Geometry: final body of the model. Coordinates: model frame, mm. Face numbers are marked on the shaded views. Round coordinates to 2 decimals unless told otherwise and drop trailing zeros. Loops run counter-clockwise (first coordinate to the right, second up) from the corner with the lowest first, then second, coordinate; pieces in that order, holes last. Notation, with made-up numbers: M 58,15 L 83,15 A31 ccw 83,52 Z; hole C 72,18.25 d11. An arc over 180 degrees is marked long. Return JSON: item names as keys, results as strings.
from build123d import *

# Parameters (mm, degrees)
CROQUIS1_R              = 32
SALIENTE_EXTRUIR1_DEPTH = 5
CROQUIS2_R              = 1.25
CORTAR_EXTRUIR1_DEPTH   = 46.530209751


with BuildPart() as part:
    # Croquis1 → Saliente-Extruir1 (new body)
    with BuildSketch(Plane.XY):
        Circle(CROQUIS1_R)
    extrude(amount=SALIENTE_EXTRUIR1_DEPTH)

    # Croquis2 → Cortar-Extruir1 (cut, through all)
    with BuildSketch(Plane.XY.offset(5)):
        with Locations((0, 28)):
            Circle(CROQUIS2_R)
        with Locations((19.798989873, 19.798989873)):
            Circle(CROQUIS2_R)
        with Locations((28, 0)):
            Circle(CROQUIS2_R)
        with Locations((19.798989873, -19.798989873)):
            Circle(CROQUIS2_R)
        with Locations((0, -28)):
            Circle(CROQUIS2_R)
        with Locations((-19.798989873, -19.798989873)):
            Circle(CROQUIS2_R)
        with Locations((-28, 0)):
            Circle(CROQUIS2_R)
        with Locations((-19.798989873, 19.798989873)):
            Circle(CROQUIS2_R)
    extrude(amount=-CORTAR_EXTRUIR1_DEPTH, mode=Mode.SUBTRACT)


solid = part.part
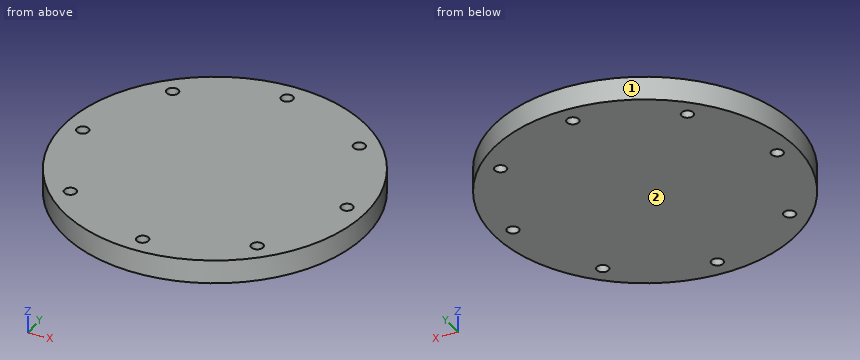
Q1. Section query D-D (x = 28). Output: boundary loops of the cut face in (y, z).
Determined:
{"outline": "M -15.49,0 L -1.25,0 L -1.25,5 L -15.49,5 Z; M 1.25,0 L 15.49,0 L 15.49,5 L 1.25,5 Z"}
Q2. Pin query (flat end, axial travel): pin 1 (2 mm diameter, centred on y = 25, z = 2, fed in from +X); pin 2 (2 mm diameter, centred on x = -22, z = 4, fed in from -Y); pin 3 (1 mm diameter, centred on x = 20, z = 2.5, fed in from -Y); pin 4 (2 mm diameter, centred on x = 28, y = 0, fed in from +Z). Return the tip coordinate at first contact, or that it passes through.
Determined:
{"pin 1": "stops at x = 21.17", "pin 2": "stops at y = -24.15", "pin 3": "stops at y = -25.37", "pin 4": "passes through"}
Q3. Section query C-C (z = 2.65). State how many separate pieces and enclosed holes the cut face has, plus the area to 3 significant figures.
Determined:
{"separate pieces": "1", "enclosed holes": "8", "area": "3,180 mm^2"}
Q4. Material intervals for L1, parallel to Y at x = 0, z = 1.1; L2, parallel to Y at x = 19, z = 4.05; L3, parallel to Y at x = -13, z = 4.1, sorted ascending.
Determined:
{"L1": "y = -32 to -29.25, -26.75 to 26.75, 29.25 to 32", "L2": "y = -25.75 to -20.76, -18.84 to 18.84, 20.76 to 25.75", "L3": "y = -29.24 to 29.24"}
Q5. Section query A-A (x = 0). Output: boundary loops of the cut face in (y, z), plus the area to 3 significant figures.
Determined:
{"outline": "M -32,0 L -29.25,0 L -29.25,5 L -32,5 Z; M -26.75,0 L 26.75,0 L 26.75,5 L -26.75,5 Z; M 29.25,0 L 32,0 L 32,5 L 29.25,5 Z", "area": "295 mm^2"}
Q6. Pull-direction query (X, two-part tool) for the marked faces 1 and 2; classes: pulls with the +X half, pulls with the -X half, needs draft (parallel to the pull), parting line crosses it, or undercut.
Determined:
{"face 1": "parting line crosses it", "face 2": "needs draft"}
